from build123d import *

# Parameters (mm, degrees)
BOSS_EXTRUDE1_DEPTH = 762
SHELL1_T            = -2


with BuildPart() as part:
    # Sketch1 → Boss-Extrude1 (new, symmetric)
    with BuildSketch(Plane(origin=(0, 0, 0), x_dir=(0, 0, -1), z_dir=(1, 0, 0))):
        with BuildLine():
            Line((-23.5, 12.5), (23.5, 12.5))
            ThreePointArc((23.5, 12.5), (24.560660172, 12.060660172), (25, 11))
            Line((25, 11), (25, -11))
            ThreePointArc((25, -11), (24.560660172, -12.060660172), (23.5, -12.5))
            Line((23.5, -12.5), (-23.5, -12.5))
            ThreePointArc((-23.5, -12.5), (-24.560660172, -12.060660172), (-25, -11))
            Line((-25, -11), (-25, 11))
            ThreePointArc((-25, 11), (-24.560660172, 12.060660172), (-23.5, 12.5))
        make_face()
    extrude(amount=BOSS_EXTRUDE1_DEPTH, both=True)

    # Shell1
    shell1_openings = [part.faces().sort_by_distance(p)[0] for p in [
        (762, 0, 0),
        (-762, 0, 0),
    ]]
    offset(amount=SHELL1_T, openings=shell1_openings, kind=Kind.INTERSECTION)

    # SurfaceCut1
    split(bisect_by=Plane(origin=(-87.5, 0, 87.5), x_dir=(0.707106781186551, 0, 0.7071067811865441), z_dir=(-0.7071067811865441, 0, 0.707106781186551)), keep=Keep.BOTTOM)

    # SurfaceCut2
    split(bisect_by=Plane(origin=(87.5, 0, 87.5), x_dir=(-0.707106781186551, 0, 0.7071067811865441), z_dir=(-0.7071067811865441, 0, -0.707106781186551)), keep=Keep.TOP)


solid = part.part
Work out the finished part from the listing and answer in its coordinate system (mm). A direction names the side the tool comes from. Coordinates: 2 decimals unless noted, no trailing zeros. Write each loop counter-clockwise with the first axis right and the second up, starting at its lowest first coordinate (ties: lowest second). Pieces come first, ordered by that corner, then holes.
1. The part is cut by section C-C, the plane y = -4.75. Write down the section's boundary in (x, z).
Results list:
outline: (-200, -25) - (200, -25) - (198, -23) - (-198, -23) - close; (-152, 23) - (152, 23) - (150, 25) - (-150, 25) - close
2. For faces 1 (the flat face through (3, 0, -25)), 2 (the flat face through (2, 0, 23)), determine the directions among +Z, -Z, +X, -X, +Y, -Y from which every point of the face is accessible in a straight line to the end or side of a thin tool.
Results list:
face 1: -Z, +X, -X, +Y, -Y
face 2: +X, -X
3. The part is cut by section A-A, the plane z = -14. Write down the section's boundary in (x, y), and give its area (3 significant figures).
Results list:
outline: (-189, -12.5) - (189, -12.5) - (189, -10.5) - (-189, -10.5) - close; (-189, 10.5) - (189, 10.5) - (189, 12.5) - (-189, 12.5) - close
area: 1,510 mm2
4. A flat-ended cylindrical pin translates along its axis: pin 1 (2 mm diameter, centred on y = 8, z = -16, fed in from -X). Find the tip coordinate at first contact, or state that the pin passes through.
Results list:
pin 1: passes through
5. The part is cut by section B-B, the plane x = -109. Write down the section's boundary in (y, z).
Results list:
outline: (-12.5, -23.5) arc R1.5 ccw to (-11, -25) - (11, -25) arc R1.5 ccw to (12.5, -23.5) - (12.5, 23.5) arc R1.5 ccw to (11, 25) - (-11, 25) arc R1.5 ccw to (-12.5, 23.5) - close; hole (-10.5, -23) - (10.5, -23) - (10.5, 23) - (-10.5, 23) - close
6. Consider line 1 along Z through (x, y) = (67.5, -3.25); line 2 along Y through (x, z) = (-74.5, -2); line 3 along Z through (x, y) = (50, 11.25). Determine where each line is inside the solid, lowest interval first.
Results list:
line 1: z = -25 to -23, 23 to 25
line 2: y = -12.5 to -10.5, 10.5 to 12.5
line 3: z = -24.98 to 24.98
